Could you check a few things on this model? Use its own coordinates, in mm. Round coordinates to 2 decimals unless told otherwise and drop trailing zeros. Loops run counter-clockwise (first coordinate to the right, second up) from the corner with the lowest first, then second, coordinate; pieces in that order, holes last. Notation, with made-up numbers: M -18.5,-14.75 L 25.5,-14.75 A20 ccw 25.5,23.25 Z; hole C 1,88.5 d7. An arc over 180 degrees is marked long. Answer in a Markdown table with one row per item.
```python
from build123d import *

# Parameters (mm, degrees)
SALIENTE_EXTRUIR1_DEPTH = 3
CORTAR_EXTRUIR1_REACH   = 5
CROQUIS2_W              = 15.3
CROQUIS2_H              = 3
CROQUIS2_W_2            = 16.15
CROQUIS2_W_3            = 3
CROQUIS2_H_2            = 44.7


with BuildPart() as part:
    # Croquis1 → Saliente-Extruir1 (new body)
    with BuildSketch(Plane.XY):
        with BuildLine():
            Line((104.8, 195), (101.5, 195))
            ThreePointArc((101.5, 195), (100.439339828, 195.439339828), (100, 196.5))
            Line((100, 196.5), (100, 250))
            Line((100, 250), (-100, 250))
            Line((-100, 250), (-100, -250))
            Line((-100, -250), (100, -250))
            Line((100, -250), (100, -35.619856886))
            Line((100, -35.619856886), (100, -30))
            Line((100, -30), (100, -5))
            Line((100, -5), (100, 68.5))
            ThreePointArc((100, 68.5), (100.439339828, 69.560660172), (101.5, 70))
            Line((101.5, 70), (112.8, 70))
            ThreePointArc((112.8, 70), (113.860660172, 70.439339828), (114.3, 71.5))
            Line((114.3, 71.5), (114.3, 108.5))
            ThreePointArc((114.3, 108.5), (113.860660172, 109.560660172), (112.8, 110))
            Line((112.8, 110), (107.8, 110))
            ThreePointArc((107.8, 110), (106.739339828, 109.560660172), (106.3, 108.5))
            Line((106.3, 108.5), (106.3, 96.5))
            ThreePointArc((106.3, 96.5), (105.860660172, 95.439339828), (104.8, 95))
            Line((104.8, 95), (101.5, 95))
            ThreePointArc((101.5, 95), (100.439339828, 95.439339828), (100, 96.5))
            Line((100, 96.5), (100, 168.5))
            ThreePointArc((100, 168.5), (100.439339828, 169.560660172), (101.5, 170))
            Line((101.5, 170), (112.8, 170))
            ThreePointArc((112.8, 170), (113.860660172, 170.439339828), (114.3, 171.5))
            Line((114.3, 171.5), (114.3, 208.5))
            ThreePointArc((114.3, 208.5), (113.860660172, 209.560660172), (112.8, 210))
            Line((112.8, 210), (107.8, 210))
            ThreePointArc((107.8, 210), (106.739339828, 209.560660172), (106.3, 208.5))
            Line((106.3, 208.5), (106.3, 196.5))
            ThreePointArc((106.3, 196.5), (105.860660172, 195.439339828), (104.8, 195))
        make_face()
    extrude(amount=SALIENTE_EXTRUIR1_DEPTH)

    # Croquis2 → Cortar-Extruir1 (cut, up to next)
    with BuildSketch(Plane.XY.offset(3), mode=Mode.PRIVATE) as cortar_extruir1_sk1:
        Polygon((-100, -250), (-80.85, -250), (-80.85, -247), (-97, -247), (-97, -202.65), (-100, -202.65), align=None)
    cortar_extruir1_tool1 = extrude(cortar_extruir1_sk1.sketch, amount=-CORTAR_EXTRUIR1_REACH, mode=Mode.PRIVATE) & part.part
    add(cortar_extruir1_tool1.solids().sort_by_distance((-99.489241, -226.325, 3))[0], mode=Mode.SUBTRACT)
    # Croquis2 → Cortar-Extruir1 (cut, up to next)
    with BuildSketch(Plane.XY.offset(3), mode=Mode.PRIVATE) as cortar_extruir1_sk2:
        with Locations((-43.5, -248.5)):
            Rectangle(CROQUIS2_W, CROQUIS2_H)
    cortar_extruir1_tool2 = extrude(cortar_extruir1_sk2.sketch, amount=-CORTAR_EXTRUIR1_REACH, mode=Mode.PRIVATE) & part.part
    add(cortar_extruir1_tool2.solids().sort_by_distance((-43.5, -248.5, 3))[0], mode=Mode.SUBTRACT)
    # Croquis2 → Cortar-Extruir1 (cut, up to next)
    with BuildSketch(Plane.XY.offset(3), mode=Mode.PRIVATE) as cortar_extruir1_sk3:
        with Locations((1.5, -248.5)):
            Rectangle(CROQUIS2_W, CROQUIS2_H)
    cortar_extruir1_tool3 = extrude(cortar_extruir1_sk3.sketch, amount=-CORTAR_EXTRUIR1_REACH, mode=Mode.PRIVATE) & part.part
    add(cortar_extruir1_tool3.solids().sort_by_distance((1.5, -248.5, 3))[0], mode=Mode.SUBTRACT)
    # Croquis2 → Cortar-Extruir1 (cut, up to next)
    with BuildSketch(Plane.XY.offset(3), mode=Mode.PRIVATE) as cortar_extruir1_sk4:
        with Locations((46.5, -248.5)):
            Rectangle(CROQUIS2_W, CROQUIS2_H)
    cortar_extruir1_tool4 = extrude(cortar_extruir1_sk4.sketch, amount=-CORTAR_EXTRUIR1_REACH, mode=Mode.PRIVATE) & part.part
    add(cortar_extruir1_tool4.solids().sort_by_distance((46.5, -248.5, 3))[0], mode=Mode.SUBTRACT)
    # Croquis2 → Cortar-Extruir1 (cut, up to next)
    with BuildSketch(Plane.XY.offset(3), mode=Mode.PRIVATE) as cortar_extruir1_sk5:
        with Locations((91.925, -248.5)):
            Rectangle(CROQUIS2_W_2, CROQUIS2_H)
    cortar_extruir1_tool5 = extrude(cortar_extruir1_sk5.sketch, amount=-CORTAR_EXTRUIR1_REACH, mode=Mode.PRIVATE) & part.part
    add(cortar_extruir1_tool5.solids().sort_by_distance((91.925, -248.5, 3))[0], mode=Mode.SUBTRACT)
    # Croquis2 → Cortar-Extruir1 (cut, up to next)
    with BuildSketch(Plane.XY.offset(3), mode=Mode.PRIVATE) as cortar_extruir1_sk6:
        with Locations((-98.5, -135)):
            Rectangle(CROQUIS2_W_3, CROQUIS2_H_2)
    cortar_extruir1_tool6 = extrude(cortar_extruir1_sk6.sketch, amount=-CORTAR_EXTRUIR1_REACH, mode=Mode.PRIVATE) & part.part
    add(cortar_extruir1_tool6.solids().sort_by_distance((-98.5, -135, 3))[0], mode=Mode.SUBTRACT)
    # Croquis2 → Cortar-Extruir1 (cut, up to next)
    with BuildSketch(Plane.XY.offset(3), mode=Mode.PRIVATE) as cortar_extruir1_sk7:
        with Locations((-98.5, -45)):
            Rectangle(CROQUIS2_W_3, CROQUIS2_H_2)
    cortar_extruir1_tool7 = extrude(cortar_extruir1_sk7.sketch, amount=-CORTAR_EXTRUIR1_REACH, mode=Mode.PRIVATE) & part.part
    add(cortar_extruir1_tool7.solids().sort_by_distance((-98.5, -45, 3))[0], mode=Mode.SUBTRACT)
    # Croquis2 → Cortar-Extruir1 (cut, up to next)
    with BuildSketch(Plane.XY.offset(3), mode=Mode.PRIVATE) as cortar_extruir1_sk8:
        with Locations((-98.5, 45)):
            Rectangle(CROQUIS2_W_3, CROQUIS2_H_2)
    cortar_extruir1_tool8 = extrude(cortar_extruir1_sk8.sketch, amount=-CORTAR_EXTRUIR1_REACH, mode=Mode.PRIVATE) & part.part
    add(cortar_extruir1_tool8.solids().sort_by_distance((-98.5, 45, 3))[0], mode=Mode.SUBTRACT)
    # Croquis2 → Cortar-Extruir1 (cut, up to next)
    with BuildSketch(Plane.XY.offset(3), mode=Mode.PRIVATE) as cortar_extruir1_sk9:
        with Locations((-98.5, 135)):
            Rectangle(CROQUIS2_W_3, CROQUIS2_H_2)
    cortar_extruir1_tool9 = extrude(cortar_extruir1_sk9.sketch, amount=-CORTAR_EXTRUIR1_REACH, mode=Mode.PRIVATE) & part.part
    add(cortar_extruir1_tool9.solids().sort_by_distance((-98.5, 135, 3))[0], mode=Mode.SUBTRACT)
    # Croquis2 → Cortar-Extruir1 (cut, up to next)
    with BuildSketch(Plane.XY.offset(3), mode=Mode.PRIVATE) as cortar_extruir1_sk10:
        Polygon((-80.85, 247), (-80.85, 250), (-100, 250), (-100, 202.65), (-97, 202.65), (-97, 247), align=None)
    cortar_extruir1_tool10 = extrude(cortar_extruir1_sk10.sketch, amount=-CORTAR_EXTRUIR1_REACH, mode=Mode.PRIVATE) & part.part
    add(cortar_extruir1_tool10.solids().sort_by_distance((-81.360759, 248.5, 3))[0], mode=Mode.SUBTRACT)
    # Croquis2 → Cortar-Extruir1 (cut, up to next)
    with BuildSketch(Plane.XY.offset(3), mode=Mode.PRIVATE) as cortar_extruir1_sk11:
        with Locations((-43.5, 248.5)):
            Rectangle(CROQUIS2_W, CROQUIS2_H)
    cortar_extruir1_tool11 = extrude(cortar_extruir1_sk11.sketch, amount=-CORTAR_EXTRUIR1_REACH, mode=Mode.PRIVATE) & part.part
    add(cortar_extruir1_tool11.solids().sort_by_distance((-43.5, 248.5, 3))[0], mode=Mode.SUBTRACT)
    # Croquis2 → Cortar-Extruir1 (cut, up to next)
    with BuildSketch(Plane.XY.offset(3), mode=Mode.PRIVATE) as cortar_extruir1_sk12:
        with BuildLine():
            ThreePointArc((41.5, 155), (59.17766953, 162.32233047), (66.5, 180))
            ThreePointArc((66.5, 180), (59.17766953, 197.67766953), (41.5, 205))
            Line((41.5, 205), (-38.5, 205))
            ThreePointArc((-38.5, 205), (-63.5, 180), (-38.5, 155))
            Line((-38.5, 155), (41.5, 155))
        make_face()
    cortar_extruir1_tool12 = extrude(cortar_extruir1_sk12.sketch, amount=-CORTAR_EXTRUIR1_REACH, mode=Mode.PRIVATE) & part.part
    add(cortar_extruir1_tool12.solids().sort_by_distance((1.5, 180, 3))[0], mode=Mode.SUBTRACT)
    # Croquis2 → Cortar-Extruir1 (cut, up to next)
    with BuildSketch(Plane.XY.offset(3), mode=Mode.PRIVATE) as cortar_extruir1_sk13:
        with Locations((46.5, 248.5)):
            Rectangle(CROQUIS2_W, CROQUIS2_H)
    cortar_extruir1_tool13 = extrude(cortar_extruir1_sk13.sketch, amount=-CORTAR_EXTRUIR1_REACH, mode=Mode.PRIVATE) & part.part
    add(cortar_extruir1_tool13.solids().sort_by_distance((46.5, 248.5, 3))[0], mode=Mode.SUBTRACT)
    # Croquis2 → Cortar-Extruir1 (cut, up to next)
    with BuildSketch(Plane.XY.offset(3), mode=Mode.PRIVATE) as cortar_extruir1_sk14:
        with Locations((1.5, 248.5)):
            Rectangle(CROQUIS2_W, CROQUIS2_H)
    cortar_extruir1_tool14 = extrude(cortar_extruir1_sk14.sketch, amount=-CORTAR_EXTRUIR1_REACH, mode=Mode.PRIVATE) & part.part
    add(cortar_extruir1_tool14.solids().sort_by_distance((1.5, 248.5, 3))[0], mode=Mode.SUBTRACT)
    # Croquis2 → Cortar-Extruir1 (cut, up to next)
    with BuildSketch(Plane.XY.offset(3), mode=Mode.PRIVATE) as cortar_extruir1_sk15:
        with Locations((91.925, 248.5)):
            Rectangle(CROQUIS2_W_2, CROQUIS2_H)
    cortar_extruir1_tool15 = extrude(cortar_extruir1_sk15.sketch, amount=-CORTAR_EXTRUIR1_REACH, mode=Mode.PRIVATE) & part.part
    add(cortar_extruir1_tool15.solids().sort_by_distance((91.925, 248.5, 3))[0], mode=Mode.SUBTRACT)
    # Croquis2 → Cortar-Extruir1 (cut, up to next)
    with BuildSketch(Plane.XY.offset(3), mode=Mode.PRIVATE) as cortar_extruir1_sk16:
        with BuildLine():
            ThreePointArc((41.5, -205), (59.17766953, -197.67766953), (66.5, -180))
            ThreePointArc((66.5, -180), (59.17766953, -162.32233047), (41.5, -155))
            Line((41.5, -155), (-38.5, -155))
            ThreePointArc((-38.5, -155), (-63.5, -180), (-38.5, -205))
            Line((-38.5, -205), (41.5, -205))
        make_face()
    cortar_extruir1_tool16 = extrude(cortar_extruir1_sk16.sketch, amount=-CORTAR_EXTRUIR1_REACH, mode=Mode.PRIVATE) & part.part
    add(cortar_extruir1_tool16.solids().sort_by_distance((1.5, -180, 3))[0], mode=Mode.SUBTRACT)


solid = part.part
```
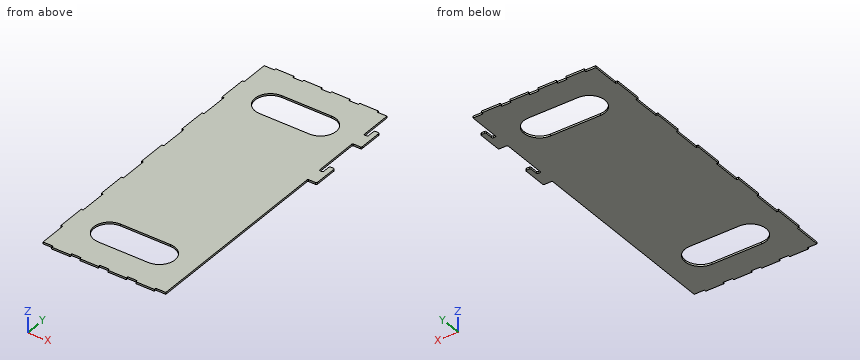
1) I want a section at D-D, the plane x = 59.5. Please give me the cut outline in (y, z), plus the area to 3 significant figures.
Computed:
| item | result |
|---|---|
| outline | M -250,0 L -197.35,0 L -197.35,3 L -250,3 Z; M -162.65,0 L 162.65,0 L 162.65,3 L -162.65,3 Z; M 197.35,0 L 250,0 L 250,3 L 197.35,3 Z |
| area | 1,290 mm² |
2) I want a section at C-C, the plane y = 3. Please give me the cut outline in (x, z).
Computed:
| item | result |
|---|---|
| outline | M -100,0 L 100,0 L 100,3 L -100,3 Z |
3) I need wall thicknesses on line 1 (Y direction, x = 40, z = 2); line 2 (Y direction, x = -16, z = 2.85); line 3 (X direction, y = 103.5, z = 0.45). Which ranges of each line are inside material? Lowest first, please.
Computed:
| item | result |
|---|---|
| line 1 | y = -247 to -205, -155 to 155, 205 to 247 |
| line 2 | y = -250 to -205, -155 to 155, 205 to 250 |
| line 3 | x = -100 to 100, 106.3 to 114.3 |
4) I want a section at A-A, the plane x = -15. Please give me the cut outline in (y, z), plus the area to 3 significant figures.
Computed:
| item | result |
|---|---|
| outline | M -250,0 L -205,0 L -205,3 L -250,3 Z; M -155,0 L 155,0 L 155,3 L -155,3 Z; M 205,0 L 250,0 L 250,3 L 205,3 Z |
| area | 1,200 mm² |
5) Will these pins go through, and if not, where does the flat tip stop? P1, Ø0.9, axis at x = 46.5, z = 1, coming from the +Y side; P2, Ø0.9, axis at x = -99, z = 1, coming from the +Y side; P3, Ø1, axis at y = 19, z = 1, coming from the +X side; P4, Ø3, axis at x = 45, y = -62, coming from the -Z side.
Computed:
| item | result |
|---|---|
| P1 | stops at y = 247 |
| P2 | stops at y = 202.65 |
| P3 | stops at x = 100 |
| P4 | stops at z = 0 |
6) I want a section at B-B, the plane z = 0.75. State how many separate pieces and enclosed holes the cut face has, plus the area to 3 significant figures.
Computed:
| item | result |
|---|---|
| separate pieces | 1 |
| enclosed holes | 2 |
| area | 87,700 mm² |
